Input: part model. Units: mm. Frame: model coordinates. A direction names the side the tool comes from. Coordinates: 2 decimals unless noted, no trailing zeros. Loops run counter-clockwise (first coordinate to the right, second up) from the corner with the lowest first, then second, coordinate; pieces in that order, holes last. Notation, with made-up numbers: (-0.5, -32) -> (6.5, -32) arc R20 cw to (6.5, -7) -> close; hole circle Ø3 at (20, 61.25). An arc over 180 degrees is marked (long way). Put each result on its own line as item: value. Start each with the question number.
1) Material intervals for L1, parallel to Z at x = -15.5, y = -42; L2, parallel to Y at x = -19.5, z = -16.5; L3, parallel to X at y = -24, z = -7, sorted ascending.
2) Set-up query: faces 5 (the cylindrical face through (-57.482, -7.129, 0.644)), 6 (the flat face through (0, 1, 31)). Return all of +Z, -Z, +X, -X, +Y, -Y with unobstructed straight access to the full face (end or side cutting, diameter ignored); none if empty.
3) Cut plane A-A (x = -18.5). Return the cut outline in (y, z), plus the area to 3 significant figures.
4) Cut plane D-D (z = 6.5). Return the cut outline in (x, y), plus the area to 3 significant figures.
5) Cut plane C-C (y = -32). Return the cut outline in (x, z).
6) Pull-direction query (Z, two-part tool) for faces 1 (the cylindrical face through (-66, -44, 0)), 2 (the cylindrical face through (-58.88, -5.7, -0.64)), 3 (the flat face through (-33, -38, 48)), 4 (the flat face through (-29, 0, 1)); classes: pulls with the +Z half, pulls with the -Z half, needs draft (parallel to the pull), parting line crosses it, or undercut.
7) Contact query for flat-ended pins moving along their axis: P1, Ø2, axis at x = -9, y = 1, coming from the +Z side; P2, Ø1.5, axis at x = -50, z = 32.5, coming from the -Y side; P3, Ø1.5, axis at x = -34.5, z = -7, coming from the -Y side; P4, Ø0.6, axis at x = -15.5, z = 47.5, coming from the +Y side. Output: stop coordinate, or through.
8) Cut plane B-B (y = -55). Return the cut outline in (x, z), plus the area to 3 significant figures.
from build123d import *

# Parameters (mm, degrees)
BOSS_EXTRUDE1_DEPTH = 46
BOSS_EXTRUDE2_START = 2
BOSS_EXTRUDE2_DEPTH = 2
FILLET1_R           = 2
CUT_EXTRUDE1_DEPTH  = 5
CUT_EXTRUDE2_DEPTH  = 141.121375957
CUT_EXTRUDE3_DEPTH  = 115.166545012
SKETCH6_R           = 2
CUT_EXTRUDE4_DEPTH  = 141.121375957


with BuildPart() as part:
    # Sketch1 → Boss-Extrude1 (new, symmetric)
    with BuildSketch(Plane.XY):
        with BuildLine():
            Line((0, 0), (-40, 0))
            ThreePointArc((-40, 0), (-57.67766953, -7.32233047), (-65, -25))
            Line((-65, -25), (-65, -77))
            Line((-65, -77), (-67, -77))
            Line((-67, -77), (-67, -25))
            ThreePointArc((-67, -25), (-59.091883092, -5.908116908), (-40, 2))
            Line((-40, 2), (0, 2))
            Line((0, 2), (0, 0))
        make_face()
    extrude(amount=BOSS_EXTRUDE1_DEPTH, both=True)

    # Sketch2 → Boss-Extrude2 (add)
    with BuildSketch(Plane.XY.offset(46).offset(BOSS_EXTRUDE2_START)):
        with BuildLine():
            Line((-67, -25), (-67, -77))
            Line((-67, -77), (0, -77))
            Line((0, -77), (0, 2))
            Line((0, 2), (-40, 2))
            ThreePointArc((-40, 2), (-59.091883092, -5.908116908), (-67, -25))
        make_face()
    boss_extrude2 = extrude(amount=-BOSS_EXTRUDE2_DEPTH)

    # Mirror1: Boss-Extrude2 across plane
    add(boss_extrude2.mirror(Plane.XY))

    # Fillet1
    fillet1_edges = [part.edges().sort_by_distance(p)[0] for p in [
        (-59.091883092, -5.908116908, 48),
        (-67, -51, 48),
        (-20, 2, 48),
        (-59.091883092, -5.908116908, -48),
        (-20, 2, -48),
        (-67, -51, -48),
    ]]
    fillet(fillet1_edges, radius=FILLET1_R)

    # Sketch3 → Cut-Extrude1 (cut)
    with BuildSketch(Plane.ZY.offset(67)):
        with BuildLine():
            Line((-3, -77), (-3, -47))
            ThreePointArc((-3, -47), (0, -44), (3, -47))
            Line((3, -47), (3, -77))
            ThreePointArc((3, -77), (0, -80), (-3, -77))
        make_face()
    extrude(amount=-CUT_EXTRUDE1_DEPTH, mode=Mode.SUBTRACT)

    # Sketch4 → Cut-Extrude2 (cut, through all)
    with BuildSketch(Plane.XY.offset(48)):
        with BuildLine():
            Line((0, -22), (-30, -22))
            ThreePointArc((-30, -22), (-32, -20), (-30, -18))
            Line((-30, -18), (0, -18))
            ThreePointArc((0, -18), (2, -20), (0, -22))
        make_face()
    extrude(amount=-CUT_EXTRUDE2_DEPTH, mode=Mode.SUBTRACT)

    # Sketch5 → Cut-Extrude3 (cut, through all)
    with BuildSketch(Plane(origin=(0, 2, 0), x_dir=(1, 0, 0), z_dir=(0, 1, 0))):
        with BuildLine():
            Line((0, -4), (-22.5, -4))
            ThreePointArc((-22.5, -4), (-29.5, 3), (-22.5, 10))
            Line((-22.5, 10), (0, 10))
            ThreePointArc((0, 10), (7, 3), (0, -4))
        make_face()
    extrude(amount=-CUT_EXTRUDE3_DEPTH, mode=Mode.SUBTRACT)

    # Sketch6 → Cut-Extrude4 (cut, through all)
    with BuildSketch(Plane.XY.offset(48)):
        with Locations((-5, -7)):
            Circle(SKETCH6_R)
        with Locations((-7, -71)):
            Circle(SKETCH6_R)
        with Locations((-58, -70)):
            Circle(SKETCH6_R)
    extrude(amount=-CUT_EXTRUDE4_DEPTH, mode=Mode.SUBTRACT)


solid = part.part
Results found:
1. L1: z = -48 to -46, 46 to 48
1. L2: y = 0 to 2
1. L3: x = -66.98 to -64.98
2. face 5: +X, -Y
2. face 6: +Z, -Z, +X, +Y, -Y
3. outline: (-77, -48) -> (-22, -48) -> (-22, -46) -> (-77, -46) -> close; (-77, 46) -> (-22, 46) -> (-22, 48) -> (-77, 48) -> close; (-18, -48) -> (0, -48) arc R2 ccw to (2, -46) -> (2, -10) -> (0, -10) -> (0, -46) -> (-18, -46) -> close; (-18, 46) -> (0, 46) -> (0, 4) -> (2, 4) -> (2, 46) arc R2 ccw to (0, 48) -> (-18, 48) -> close
3. area: 454 mm2
4. outline: (-67, -77) -> (-65, -77) -> (-65, -25) arc R25 cw to (-40, 0) -> (0, 0) -> (0, 2) -> (-40, 2) arc R27 ccw to (-67, -25) -> close
4. area: 266 mm2
5. outline: (-67, -46) arc R2 ccw to (-65, -48) -> (0, -48) -> (0, -46) -> (-65, -46) -> (-65, 46) -> (0, 46) -> (0, 48) -> (-65, 48) arc R2 ccw to (-67, 46) -> close
6. face 1: undercut
6. face 2: needs draft
6. face 3: pulls with the +Z half
6. face 4: undercut
7. P1: stops at z = 48
7. P2: stops at y = -2.43
7. P3: stops at y = 0
7. P4: stops at y = 1.6
8. outline: (-67, -46) arc R2 ccw to (-65, -48) -> (0, -48) -> (0, -46) -> (-65, -46) -> (-65, -3) -> (-67, -3) -> close; (-67, 3) -> (-65, 3) -> (-65, 46) -> (0, 46) -> (0, 48) -> (-65, 48) arc R2 ccw to (-67, 46) -> close
8. area: 438 mm2
